Could you check a few things on this drawing? It's one solid part, dimensions in mm from its lowest x, y, z. A direction names the side the tool comes from. Coordinates: 2 decimals unless noted, no trailing zeros. Order: outer loops, then holes, each group sorted by start corner. A loop starts at its lowest first (then second) coordinate and runs counter-clockwise, first axis right, second up.
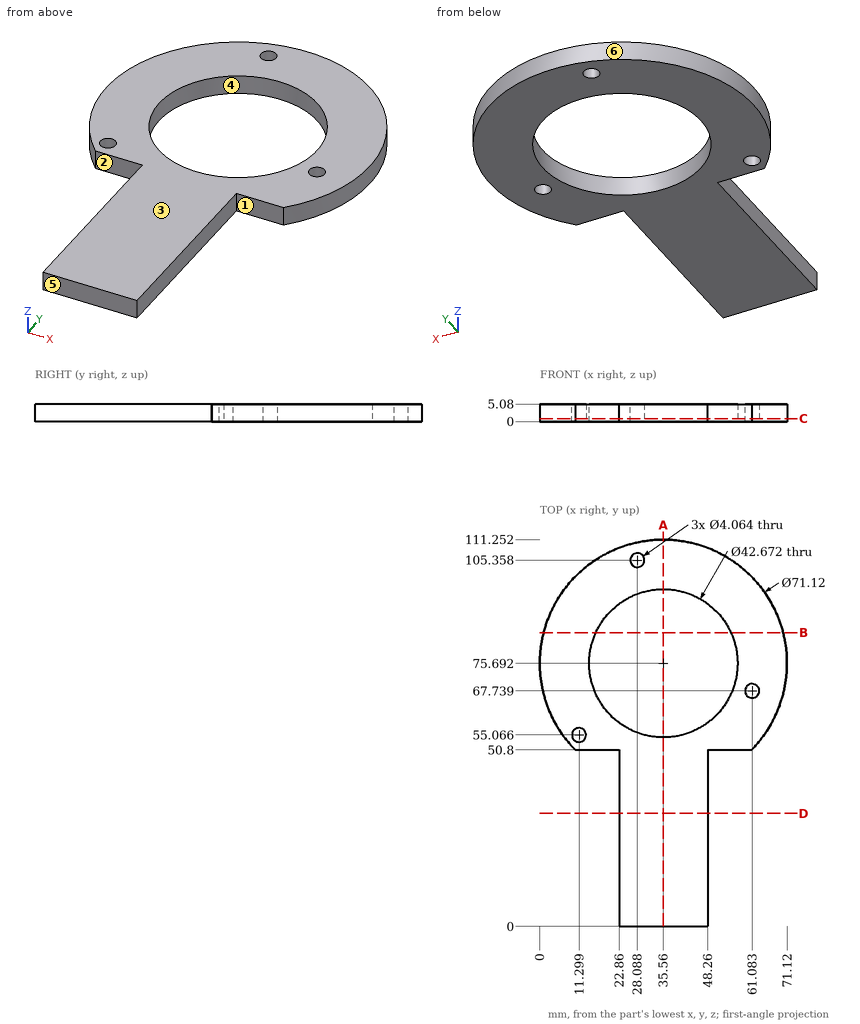
Q1. We'd pull the mould along X, two halves only. Please class the marked faces 4, 5 and 6: pulls with the +X half, pulls with the -X half, needs draft (parallel to the pull), parting line crosses it, or undercut.
Q2. Will these pins go through, and if not, where does the flat tip stop? pin 1 (3.5 mm diameter, centred on x = 61.08, y = 67.74, fed in from -Z); pin 2 (1.5 mm diameter, centred on y = 28, z = 1.5, fed in from -X); pin 3 (2.5 mm diameter, centred on x = 52.5, z = 2.5, fed in from -Y); pin 4 (2.5 mm diameter, centred on y = 20.5, z = 2, fed in from +X).
Q3. If we section it at D-D on y = 32.5: Write out the boundary of the cut face in (x, z).
Q4. For the marked faces 1, 2 and 3, which set-ups out of +Z, -Z, +X, -X, +Y, -Y let a thin tool reach every point of the face, with its end or its side?
Q5. If we section it at B-B on y = 84.5: Write out the boundary of the cut face in (x, z).
Q6. If we section it at C-C on z = 0.9: Write out the boundary of the cut face in (x, y) (1 decimal), then the cut area to 3 significant figures.
Q7. I need wall thicknesses on L1, parallel to Y at x = 29, z = 4.35 (1 decimal); L2, parallel to X at y = 66.5, z = 3.25 (1 decimal); L3, parallel to X at y = 42.5, z = 3.85. Which ranges of each line are inside material? Lowest first, please.
Q8. If we section it at A-A on x = 35.56: Write out the boundary of the cut face in (y, z).
Reply:
1. face 4: undercut
1. face 5: needs draft
1. face 6: parting line crosses it
2. pin 1: passes through
2. pin 2: stops at x = 22.86
2. pin 3: stops at y = 50.8
2. pin 4: stops at x = 48.26
3. outline: (22.86, 0) - (48.26, 0) - (48.26, 5.08) - (22.86, 5.08) - close
4. face 1: +Z, -Z, +X, -Y
4. face 2: +Z, -Z, -X, -Y
4. face 3: +Z, +X, -X, +Y, -Y
5. outline: (1.11, 0) - (16.13, 0) - (16.13, 5.08) - (1.11, 5.08) - close; (54.99, 0) - (70.01, 0) - (70.01, 5.08) - (54.99, 5.08) - close
6. outline: (10.2, 50.8) - (22.9, 50.8) - (22.9, 0) - (48.3, 0) - (48.3, 50.8) - (61, 50.8) arc R35.6 ccw (long way) to start; hole circle Ø4.1 at (11.3, 55.1); hole circle Ø42.7 at (35.6, 75.7); hole circle Ø4.1 at (28.1, 105.4); hole circle Ø4.1 at (61.1, 67.7)
6. area: 3,420 mm2
7. L1: y = 0 to 55.4, 96 to 103.5, 107.2 to 110.6
7. L2: x = 1.2 to 16.3, 54.8 to 59.5, 62.7 to 69.9
7. L3: x = 22.86 to 48.26
8. outline: (0, 0) - (54.36, 0) - (54.36, 5.08) - (0, 5.08) - close; (97.03, 0) - (111.25, 0) - (111.25, 5.08) - (97.03, 5.08) - close
